from build123d import *

# Parameters (mm, degrees)
BOSS_EXTRUDE1_DEPTH            = 5
M6_CLEARANCE_HOLE1_D           = 6.6
M6_CLEARANCE_HOLE1_CSINK_D     = 6.65
M6_CLEARANCE_HOLE1_CSINK_ANGLE = 90


with BuildPart() as part:
    # Sketch1 → Boss-Extrude1 (new body)
    with BuildSketch(Plane.XY):
        with BuildLine():
            Line((-37.5, 22.9169235), (-37.5, 60.9169235))
            Line((-37.5, 60.9169235), (-37.5, 100.9169235))
            Line((-37.5, 100.9169235), (37.5, 100.9169235))
            Line((37.5, 100.9169235), (37.5, 60.9169235))
            Line((37.5, 60.9169235), (37.5, 22.9169235))
            Line((37.5, 22.9169235), (29.682732645, 22.9169235))
            ThreePointArc((29.682732645, 22.9169235), (0, 37.5), (-29.682732645, 22.9169235))
            Line((-29.682732645, 22.9169235), (-37.5, 22.9169235))
        make_face()
    extrude(amount=BOSS_EXTRUDE1_DEPTH)

    # M6 Clearance Hole1 (through all)
    with Locations(Plane(origin=(0, 0, 0), x_dir=(-1, 0, 0), z_dir=(0, 0, -1))):
        with Locations((-22.5, 45.9169235), (22.5, 45.9169235), (22.5, 85.9169235), (-22.5, 85.9169235)):
            CounterSinkHole(M6_CLEARANCE_HOLE1_D / 2, M6_CLEARANCE_HOLE1_CSINK_D / 2, counter_sink_angle=M6_CLEARANCE_HOLE1_CSINK_ANGLE)


solid = part.part
Design review of the part built by this model. Coordinates are the model's own, in mm. Round coordinates to 2 decimals unless told otherwise and drop trailing zeros. Write each loop counter-clockwise with the first axis right and the second up, starting at its lowest first coordinate (ties: lowest second). Pieces come first, ordered by that corner, then holes. Notation, with made-up numbers: (-8.75, 27.5) - (48.25, 27.5) arc R24 cw to (48.25, 43.5) - close; hole circle Ø2 at (57.25, 4). An arc over 180 degrees is marked (long way). Return JSON: item names as keys, results as strings. Group by question number.
Item 1: The part is to be moulded in two halves that separate along X. For faces 1 (the face through (24.27, 88.7, 2.55)), 2 (the face through (-34, 22.917, 2)), 3 (the face through (0.479, 37.497, 2.465)), 4 (the face through (37.5, 62, 2)), say which applies: pulls with the +X half, pulls with the -X half, needs draft (parallel to the pull), parting line crosses it, or undercut.
Item 2: We need section C-C on y = 84. Give the number of separate pieces and of enclosed holes in the cut face, and give its area (3 significant figures).
Item 3: We need section B-B on z = 3.35. Write out the cut boundary in (x, y).
Item 4: For probe 1 along X at (y, z) = (43.5, 3); probe 2 along Y at (x, z) = (22.5, 3.55); probe 3 along Y at (x, z) = (23.5, 2.05), list the stretches that pass through material, from the lowest coordinate up. Write a range as [from, to].
Item 5: We need section A-A on x = -22.5. Write out the cut boundary in (y, z) (3 decimals).
Item 6: We need section D-D on x = 13.5. Write out the cut boundary in (y, z), and give its area (3 significant figures).
Model answer:
{
 "1": {"face 1": "undercut", "face 2": "needs draft", "face 3": "undercut", "face 4": "pulls with the +X half"},
 "2": {"separate pieces": "3", "enclosed holes": "0", "area": "321 mm²"},
 "3": {"outline": "(-37.5, 22.92) - (-29.68, 22.92) arc R37.5 cw to (29.68, 22.92) - (37.5, 22.92) - (37.5, 100.92) - (-37.5, 100.92) - close; hole circle Ø6.6 at (-22.5, 45.92); hole circle Ø6.6 at (-22.5, 85.92); hole circle Ø6.6 at (22.5, 45.92); hole circle Ø6.6 at (22.5, 85.92)"},
 "4": {"probe 1": "x = [-37.5, -24.75], [-20.25, 20.25], [24.75, 37.5]", "probe 2": "y = [30, 42.62], [49.22, 82.62], [89.22, 100.92]", "probe 3": "y = [29.22, 42.77], [49.06, 82.77], [89.06, 100.92]"},
 "5": {"outline": "(30, 0) - (42.592, 0) - (42.617, 0.025) - (42.617, 5) - (30, 5) - close; (49.217, 0.025) - (49.242, 0) - (82.592, 0) - (82.617, 0.025) - (82.617, 5) - (49.217, 5) - close; (89.217, 0.025) - (89.242, 0) - (100.917, 0) - (100.917, 5) - (89.217, 5) - close"},
 "6": {"outline": "(34.99, 0) - (100.92, 0) - (100.92, 5) - (34.99, 5) - close", "area": "330 mm²"}
}
